from build123d import *

# Parameters (mm, degrees)
SKETCH1_W           = 76.2
SKETCH1_H           = 12.7
BOSS_EXTRUDE1_DEPTH = 50.8
SKETCH3_R           = 1.0922
SKETCH3_R_2         = 2.921
CUT_EXTRUDE2_DEPTH  = 93.457395594
FILLET1_R           = 10.16
CHAMFER1_SIZE       = 1.5875


with BuildPart() as part:
    # Sketch1 → Boss-Extrude1 (new body)
    with BuildSketch(Plane(origin=(0, 0, 0), x_dir=(0, 0, -1), z_dir=(1, 0, 0))):
        with Locations((38.1, 6.35)):
            Rectangle(SKETCH1_W, SKETCH1_H)
    extrude(amount=BOSS_EXTRUDE1_DEPTH)

    # Sketch3 → Cut-Extrude2 (cut, through all)
    with BuildSketch(Plane.XZ):
        with Locations(Location((13.9065, -25.4, 0), (0, 0, 270))):
            Circle(SKETCH3_R)
        with Locations(Location((25.4, -63.5, 0), (0, 0, 270))):
            Circle(SKETCH3_R_2)
        with Locations(Location((25.4, -12.7, 0), (0, 0, 270))):
            Circle(SKETCH3_R_2)
        with Locations(Location((3.4925, -25.4, 0), (0, 0, 270))):
            Circle(SKETCH3_R)
        with Locations(Location((3.4925, -47.5996, 0), (0, 0, 270))):
            Circle(SKETCH3_R)
        with Locations(Location((13.9065, -47.5996, 0), (0, 0, 270))):
            Circle(SKETCH3_R)
    extrude(amount=-CUT_EXTRUDE2_DEPTH, mode=Mode.SUBTRACT)

    # Fillet1
    fillet1_edges = [part.edges().sort_by_distance(p)[0] for p in [
        (50.8, 6.35, -76.2),
        (50.8, 6.35, 0),
        (0, 6.35, -76.2),
        (0, 6.35, 0),
    ]]
    fillet(fillet1_edges, radius=FILLET1_R)

    # Chamfer1
    chamfer1_edges = [part.edges().sort_by_distance(p)[0] for p in [
        (25.4, 12.7, 0),
        (0, 12.7, -38.1),
        (50.8, 12.7, -38.1),
        (25.4, 12.7, -76.2),
        (47.824204897, 12.7, -73.224204897),
        (2.975795103, 12.7, -73.224204897),
        (47.824204897, 12.7, -2.975795103),
        (2.975795103, 12.7, -2.975795103),
    ]]
    chamfer(chamfer1_edges, length=CHAMFER1_SIZE)


solid = part.part
Here's how the part is built. I have some questions about the finished solid (model axes, mm). Round coordinates to 2 decimals unless told otherwise and drop trailing zeros. Write each loop counter-clockwise with the first axis right and the second up, starting at its lowest first coordinate (ties: lowest second). Pieces come first, ordered by that corner, then holes.
1. If we mould it in two halves opening along X, with no side actions, what happens to faces 1 (the conical face through (46.95, 12.45, -72.21)), 2 (the cylindrical face through (3.82, 6.26, -48.64)), 3 (the cylindrical face through (3.055, 5.634, -2.897))? For each: released by +X, released by -X, zero draft, split by the parting line, or undercut.
2. Will this pin go through, and if not, where does the flat tip stop? pin 1 Ø1.5 at (x, z) = (40, -34.5) entering from -Y.
3. Suppose I cut it at D-D (y = 10). List the corners of the cut face in (x, z) for me.
4. Suppose I cut it at B-B (x = 25.4). List the corners of the cut face in (y, z) for me, and give its area (3 significant figures).
5. Suppose I cut it at C-C (z = -63.5). List the corners of the cut face in (x, y) for me.
6. Suppose I cut it at A-A (z = -25.4). List the corners of the cut face in (x, y) for me, and give its area (3 significant figures).
7. I need wall thicknesses on L1, parallel to X at y = 3, z = -25.4; L2, parallel to Z at x = 13.5, y = 7.5; L3, parallel to Z at x = 26.5, y = 6.75. Which ranges of each line are inside material? Lowest first, please.
Answer sheet:
1. face 1: released by +X
1. face 2: undercut
1. face 3: released by -X
2. pin 1: stops at y = 0
3. outline: (0, -66.04) arc R10.16 ccw to (10.16, -76.2) - (40.64, -76.2) arc R10.16 ccw to (50.8, -66.04) - (50.8, -10.16) arc R10.16 ccw to (40.64, 0) - (10.16, 0) arc R10.16 ccw to (0, -10.16) - close; hole circle Ø2.18 at (3.49, -47.6); hole circle Ø2.18 at (3.49, -25.4); hole circle Ø2.18 at (13.91, -47.6); hole circle Ø2.18 at (13.91, -25.4); hole circle Ø5.84 at (25.4, -63.5); hole circle Ø5.84 at (25.4, -12.7)
4. outline: (0, -76.2) - (11.11, -76.2) - (12.7, -74.61) - (12.7, -66.42) - (0, -66.42) - close; (0, -60.58) - (12.7, -60.58) - (12.7, -15.62) - (0, -15.62) - close; (0, -9.78) - (12.7, -9.78) - (12.7, -1.59) - (11.11, 0) - (0, 0) - close
4. area: 817 mm2
5. outline: (0, 0) - (22.48, 0) - (22.48, 12.7) - (1.59, 12.7) - (0, 11.11) - close; (28.32, 0) - (50.8, 0) - (50.8, 11.11) - (49.21, 12.7) - (28.32, 12.7) - close
6. outline: (0, 0) - (2.4, 0) - (2.4, 12.7) - (1.59, 12.7) - (0, 11.11) - close; (4.58, 0) - (12.81, 0) - (12.81, 12.7) - (4.58, 12.7) - close; (15, 0) - (50.8, 0) - (50.8, 11.11) - (49.21, 12.7) - (15, 12.7) - close
6. area: 587 mm2
7. L1: x = 0 to 2.4, 4.58 to 12.81, 15 to 50.8
7. L2: z = -76.2 to -48.61, -46.59 to -26.41, -24.39 to 0
7. L3: z = -76.2 to -66.21, -60.79 to -15.41, -9.99 to 0
